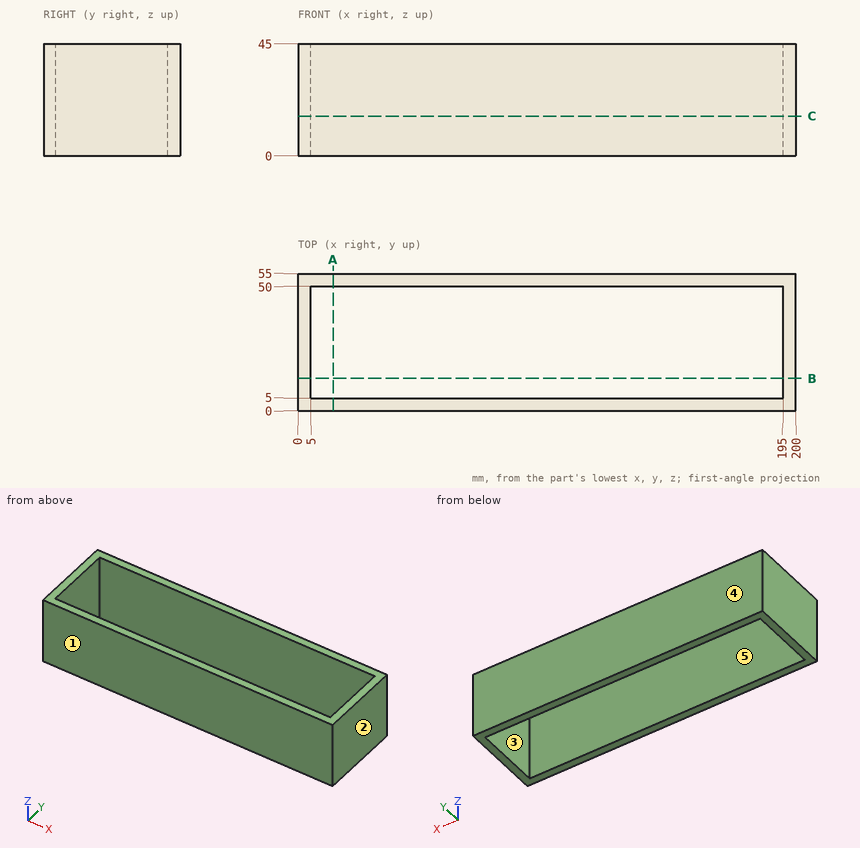
Here's the drawing with two shaded views (mm, measured from the low corner). I have some questions. A direction names the side the tool comes from. Give positions to 0.01 mm unless a question says otherwise; leave off trailing zeros. Write each loop counter-clockwise with the first axis right and the second up, starting at its lowest first coordinate (ties: lowest second). Pieces come first, ordered by that corner, then holes. Notation, with made-up numbers: (-10, 75) -> (26, 75) arc R36 cw to (26, 112) -> close; hole circle Ø4 at (-18, -36). An arc over 180 degrees is marked (long way). One line per item, written item: value.
Q1. We'd pull the mould along X, two halves only. Please class the marked faces 1, 2 and 3: +X half, -X half, draft (parallel to the pull), parting line (faces both ways), or undercut.
Results found:
face 1: draft
face 2: +X half
face 3: undercut
Q2. Imagine slicing it at A-A on x = 14. Please give me the cut outline in (y, z), and give its area (3 significant figures).
Results found:
outline: (0, 0) -> (5, 0) -> (5, 45) -> (0, 45) -> close; (50, 0) -> (55, 0) -> (55, 45) -> (50, 45) -> close
area: 450 mm^2
Q3. Which directions (+Z, -Z, +X, -X, +Y, -Y) give clear straight access to the entire face, cutting with the end or side of a thin tool? Please do the marked faces 4 and 5.
Results found:
face 4: +Z, -Z, +X, -X, +Y
face 5: +Z, -Z
Q4. Please list where these lines run through material, in increasing order: line 1 (Y direction, x = 68, z = 3); line 2 (X direction, y = 18, z = 39.5). Write a range as [from, to].
Results found:
line 1: y = [0, 5], [50, 55]
line 2: x = [0, 5], [195, 200]
Q5. Imagine slicing it at C-C on z = 16. Please give me the cut outline in (x, y), and give its area (3 significant figures).
Results found:
outline: (0, 0) -> (200, 0) -> (200, 55) -> (0, 55) -> close; hole (5, 5) -> (195, 5) -> (195, 50) -> (5, 50) -> close
area: 2,450 mm^2
Q6. Imagine slicing it at B-B on y = 13. Please give me the cut outline in (x, z), and give its area (3 significant figures).
Results found:
outline: (0, 0) -> (5, 0) -> (5, 45) -> (0, 45) -> close; (195, 0) -> (200, 0) -> (200, 45) -> (195, 45) -> close
area: 450 mm^2
